The listing builds one solid part. Answer for the finished solid, in the listing's coordinates (mm). Face numbers are marked on the shaded views. Give positions to 0.01 mm unless a question says otherwise; leave off trailing zeros. Order: outer loops, then holes, each group sorted by start corner. A loop starts at its lowest first (then second) coordinate and runs counter-clockwise, first axis right, second up. Notation, with made-up numbers: (37.5, -4.5) - (75.5, -4.5) arc R21 ccw to (75.5, 20.5) - close; hole circle Ø2 at (7.25, -27). An arc over 180 degrees is marked (long way). Write each question's results on one line, items separated by ' | '. Start each with the question number.
1. Section C-C (y = 5) is taken. Give the vertices of the cut face in (x, z) (3 decimals).
2. Determine the mould class of the marked faces 1 and 2 for opening direction X: released by +X, released by -X, zero draft, split by the parting line, or undercut.
3. Section D-D (y = 18) is taken. Give the vertices of the cut face in (x, z).
4. Find the intervals of material crossed by L1, parallel to X at y = 11.5, z = 10.25; L2, parallel to Z at x = 78, y = 0; L3, parallel to Z at x = 34.5, y = -22, in increasing order.
5. Section B-B (z = 15) is taken. Give the vertices of the cut face in (x, y).
6. Flat-ended cylindrical pins translate along their axes: pin 1 (5 mm diameter, centred on x = -72.5, z = 18, fed in from +Y); pin 2 (12.5 mm diameter, centred on y = -4.5, z = 14, fed in from +X); pin 3 (3 mm diameter, centred on x = -77, z = 22, fed in from -Y); pin 4 (4 mm diameter, centred on x = -40.5, y = 3, fed in from -Z). Find the tip coordinate at first contact, or state that the pin passes through.
7. Section A-A (z = 24.75) is taken. Give the vertices of the cut face in (x, y).
from build123d import *

# Parameters (mm, degrees)
SKETCH_W     = 180
SKETCH_H     = 100
PAD_DEPTH    = 5
SKETCH001_W  = 10
SKETCH001_H  = 40
PAD001_DEPTH = 25
SKETCH002_R  = 8
POCKET_DEPTH = 170.001


with BuildPart() as part:
    # Sketch → Pad (new body)
    with BuildSketch(Plane.XY):
        Rectangle(SKETCH_W, SKETCH_H)
    extrude(amount=PAD_DEPTH)

    # Sketch001 → Pad001 (new body)
    with BuildSketch(Plane.XY.offset(5)):
        with Locations((-75, 0)):
            Rectangle(SKETCH001_W, SKETCH001_H)
    pad001 = extrude(amount=PAD001_DEPTH)

    # Mirrored: Pad001 across Sketch001 V_Axis
    add(pad001.mirror(Plane(origin=(0, 0, 5), x_dir=(0, 0, 1), z_dir=(1, 0, 0))))

    # Sketch002 → Pocket (cut, through all)
    with BuildSketch(Plane(origin=(-80, 0, 0), x_dir=(0, -1, 0), z_dir=(-1, 0, 0))):
        with Locations((0, 15)):
            Circle(SKETCH002_R)
    extrude(amount=-POCKET_DEPTH, mode=Mode.SUBTRACT)


solid = part.part
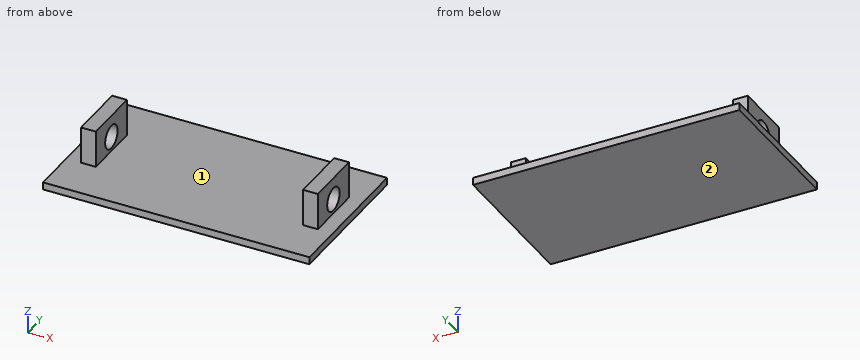
Reported:
1) outline: (-90, 0) - (90, 0) - (90, 5) - (80, 5) - (80, 8.755) - (70, 8.755) - (70, 5) - (-70, 5) - (-70, 8.755) - (-80, 8.755) - (-80, 5) - (-90, 5) - close; (-80, 21.245) - (-70, 21.245) - (-70, 30) - (-80, 30) - close; (70, 21.245) - (80, 21.245) - (80, 30) - (70, 30) - close
2) face 1: undercut | face 2: zero draft
3) outline: (-90, 0) - (90, 0) - (90, 5) - (80, 5) - (80, 30) - (70, 30) - (70, 5) - (-70, 5) - (-70, 30) - (-80, 30) - (-80, 5) - (-90, 5) - close
4) L1: -80 to -70, 70 to 80 | L2: 0 to 7, 23 to 30 | L3: 0 to 5
5) outline: (-80, -20) - (-70, -20) - (-70, -8) - (-80, -8) - close; (-80, 8) - (-70, 8) - (-70, 20) - (-80, 20) - close; (70, -20) - (80, -20) - (80, -8) - (70, -8) - close; (70, 8) - (80, 8) - (80, 20) - (70, 20) - close
6) pin 1: y = 20 | pin 2: x = 80 | pin 3: y = -20 | pin 4: z = 0
7) outline: (-80, -20) - (-70, -20) - (-70, 20) - (-80, 20) - close; (70, -20) - (80, -20) - (80, 20) - (70, 20) - close
